Geometry: final body of the model. Coordinates: model frame, mm. Face numbers are marked on the shaded views. A direction names the side the tool comes from. Give positions to 0.01 mm unless a question says otherwise; leave off trailing zeros. Write each loop counter-clockwise with the first axis right and the second up, starting at its lowest first coordinate (ties: lowest second). Pieces come first, ordered by that corner, then holes. Notation, with made-up numbers: (64.25, -5) - (111.25, -5) arc R15 ccw to (111.25, 7) - close; hole circle Ø2 at (-9, 27). An arc over 180 degrees is marked (long way). Use CSV: the item, a comma, the result in double quotes. Start each with the question number.
(1) Reachability of the marked faces 4, 5, 6 and 7 from +Z, -Z, +X, -X, +Y, -Y: full face, straight path, thin tool, end or side. Return the list, or none.
(2) Section C-C on x = -4.5. Output: boundary loops of the cut face in (y, z), and give its area (3 significant figures).
(3) First-contact query: pin 1 Ø10 at (x, z) = (10.5, -15.5) entering from -Y; pin 2 Ø1.5 at (x, y) = (11.5, -3.5) entering from +Z; pin 3 Ø1.5 at (y, z) = (-17, -28) entering from +X. Flat tips, straight axial feed; report the tip coordinate or a pass-through.
(4) Draft query along X for the marked faces 1, 2 and 3. Return one class per face: released by +X, released by -X, zero draft, split by the parting line, or undercut.
(5) Line query: probe 1 along X at (y, z) = (-15, -26); probe 2 along Y at (x, z) = (7, -0.5); probe 3 along Z at (x, y) = (-0.5, -0.5). Output: solid intervals per line, ascending. Write a range as [from, to].
(6) Section B-B on y = -8. Output: boundary loops of the cut face in (x, z), and give its area (3 significant figures).
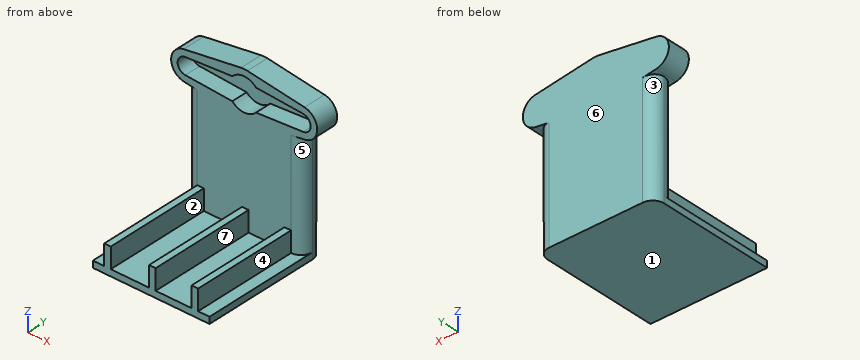
Autodesk Fusion 360 part; units mm, degrees
sketch "Sketch1" plane through (0, 0, 0) normal (0, 1, 0) x (1, 0, 0)
  line L0 (0, 0) -> (16.3, 0) construction
  line L1 (2.9047, 2.75) -> (2.9047, -2.75) construction
  line L2 (2.9047, 2.75) -> (14.4306, 1.9957)
  line L3 (2.9047, -2.75) -> (14.4306, -1.9957)
  line L4 (0, 4) -> (0, -4) construction
  arc A0 (14.4306, -1.9957) -> (14.4306, 1.9957) centre (14.3, 0) ccw
  line L5 (0.7832, 5.545) -> (14.8035, 3.5646)
  line L6 (0.7832, -5.545) -> (14.8035, -3.5646)
  arc A1 (14.8035, -3.5646) -> (14.8035, 3.5646) centre (14.3, 0) ccw
  line L7 (-2.9047, 2.75) -> (-14.4306, 1.9957)
  line L8 (-0.7832, 5.545) -> (-14.8035, 3.5646)
  line L9 (-2.9047, -2.75) -> (-14.4306, -1.9957)
  line L10 (-0.7832, -5.545) -> (-14.8035, -3.5646)
  arc A2 (-14.4306, 1.9957) -> (-14.4306, -1.9957) centre (-14.3, 0) ccw
  arc A3 (-14.8035, 3.5646) -> (-14.8035, -3.5646) centre (-14.3, 0) ccw
  arc A4 (0.7832, 5.545) -> (-0.7832, 5.545) centre (0, 0) ccw
  arc A5 (-0.7832, -5.545) -> (0.7832, -5.545) centre (0, 0) ccw
  arc A6 (2.9047, 2.75) -> (-2.9047, 2.75) centre (0, 0) ccw
  arc A7 (-2.9047, -2.75) -> (2.9047, -2.75) centre (0, 0) ccw
  line L11 (14.3, 3.6357) -> (14.3, 31.6)
  line L12 (14.3, 30) -> (-14.3, 30)
  line L13 (-14.3, 30) -> (-14.3, 3.6357)
  line L14 (14.3, 31.6) -> (-14.3, 31.6)
  line L15 (-14.3, 31.6) -> (-14.3, 30)
  dimension "d1" = 8
  dimension "d2" = 16.3
  dimension "d3" = 4
  dimension "d5" = 5.5
  dimension "d6" = 1.6
  dimension "d7" = 1.6
  dimension "d8" = 30
  dimension "d16" = 1.6
extrude "Extrude1" add sketch "Sketch1" along normal blind 1.6 contours L2 L3 A0 L7 L9 A2 A6 A7 | L5 L8 A4 L11 L12 L13 | L5 L6 A1 L8 L10 A3 A4 A5 | L11 L12 L14 L15
extrude "Extrude2" add sketch "Sketch1" against normal blind 4 contours L5 L8 A4 L11 L12 L13 | L5 L6 A1 L8 L10 A3 A4 A5
extrude "Extrude3" add sketch "Sketch1" against normal blind 30 contours L11 L12 L14 L15
fillet "Fillet1" radius 2.8 4 edges at (14.3, 1.6, -17.6179) (14.3, -4, -16.8179) (-14.3, 1.6, -17.6179) (-14.3, -4, -16.8179)
ref_plane "WorkPlane1" through (0.3, -15.6, -30.8) normal (1, 0, 0) x (0, 0, -1)
ref_plane "WorkPlane2" through (-11.5, -15.6, -30.8) normal (-1, 0, 0) x (0, 0, 1)
ref_plane "WorkPlane3" through (11.5, -15.6, -30.8) normal (1, 0, 0) x (0, 0, -1)
sketch "Sketch2" plane through (0.3, -15.6, -30.8) normal (1, 0, 0) x (0, 0, -1)
  line L0 (-0.8, 14.4) -> (-0.8, -14.4)
  line L1 (-0.8, -14.4) -> (-5.8, -14.4)
  line L2 (-5.8, -14.4) -> (-5.8, 11.6)
  line L3 (-5.8, 11.6) -> (-0.8, 11.6)
  line L4 (-0.8, 11.6) -> (-0.8, -14.4)
  line L5 (-26.7688, 11.6) -> (-0.8, 11.6)
  dimension "d25" = 5
sketch "Sketch3" plane through (-11.5, -15.6, -30.8) normal (-1, 0, 0) x (0, 0, -1)
  line L0 (-5.8, 14.4) -> (-5.8, -11.6)
  line L1 (-0.8, 14.4) -> (-5.8, 14.4)
  line L2 (-0.8, -11.6) -> (-0.8, 14.4)
  line L3 (-5.8, -11.6) -> (-0.8, -11.6)
sketch "Sketch4" plane through (11.5, -15.6, -30.8) normal (1, 0, 0) x (0, 0, -1)
  line L0 (-5.8, -14.4) -> (-5.8, 11.6)
  line L1 (-0.8, -14.4) -> (-5.8, -14.4)
  line L2 (-0.8, 11.6) -> (-0.8, -14.4)
  line L3 (-5.8, 11.6) -> (-0.8, 11.6)
extrude "Extrude4" add sketch "Sketch2" along normal mid plane 1.6
extrude "Extrude5" add sketch "Sketch4" against normal blind 1.6
extrude "Extrude6" add sketch "Sketch3" against normal blind 1.6
equation "d7 = d6"
Check values:
1,face 4,"+Z, +X, -Y"
1,face 5,"+X, -Y"
1,face 6,"+Z, -Z, +X, -X, +Y"
1,face 7,"+Z, -Y"
2,outline,"(-30, -31.6) - (1.6, -31.6) - (1.6, 5.02) - (-4, 5.02) - (-4, 2.65) - (0, 2.65) - (0, -2.65) - (-4, -2.65) - (-4, -30) - (-30, -30) - close"
2,area,"226 mm²"
3,pin 1,"stops at y = -4"
3,pin 2,"stops at z = 4.14"
3,pin 3,"stops at x = 11.5"
4,face 1,"zero draft"
4,face 2,"undercut"
4,face 3,"released by -X"
5,probe 1,"x = [-11.5, -9.9], [-0.5, 1.1], [9.9, 11.5]"
5,probe 2,"y = [0, 1.6]"
5,probe 3,"z = [-31.6, -3.97], [3.97, 5.58]"
6,outline,"(-14.3, -31.6) - (14.3, -31.6) - (14.3, -30) - (11.5, -30) - (11.5, -25) - (9.9, -25) - (9.9, -30) - (1.1, -30) - (1.1, -25) - (-0.5, -25) - (-0.5, -30) - (-9.9, -30) - (-9.9, -25) - (-11.5, -25) - (-11.5, -30) - (-14.3, -30) - close"
6,area,"69.8 mm²"
